Read the model definition and answer for the solid it produces. Units are mm, in the model's axes. A direction names the side the tool comes from. Coordinates: 2 decimals unless noted, no trailing zeros. Loops run counter-clockwise (first coordinate to the right, second up) from the corner with the lowest first, then second, coordinate; pieces in that order, holes last. Notation, with made-up numbers: M 65.5,84 L 104.5,84 A33 ccw 104.5,119 Z; hole C -13,8 d9. An arc over 180 degrees is marked long. One line per item, written item: value. Start each with the question number.
1. For faces 4 (the face through (-12.46, -83, 15)), 5 (the face through (13, -42, 30)), 6 (the face through (-15, -86, 15)), determine the directions among +Z, -Z, +X, -X, +Y, -Y from which every point of the face is accessible in a straight line to the end or side of a thin tool.
2. Flat-ended cylindrical pins translate along their axes: pin 1 (10 mm diameter, centred on x = -25.5, z = 20.5, fed in from -Y); pin 2 (3 mm diameter, centred on x = 19.5, z = 27, fed in from +Y); pin 3 (12.5 mm diameter, centred on x = -1.5, z = 9.5, fed in from +Y); pin 4 (5 mm diameter, centred on x = 32, z = 11.5, fed in from -Y). Find the tip coordinate at first contact, or state that the pin passes through.
3. The part is cut by section C-C (z = 6.75). Write down the section's boundary in (x, y), then the cut area to 3 significant figures.
4. The part is cut by section A-A (x = 0). Write down the section's boundary in (y, z), then the cut area to 3 significant figures.
5. The part is cut by section B-B (y = 0). Write down the section's boundary in (x, z), then the cut area to 3 significant figures.
6. Consider probe 1 along X at (y, z) = (0, 22); probe 2 along X at (y, z) = (-96, 3); probe 3 along Y at (x, z) = (6, 24.25). Determine where each line is inside the solid, lowest interval first.
7. Determine the mould class of faces 1 (the face through (0, -129.31, 15)), 2 (the face through (0, -126.77, 15)), 3 (the face through (15, -87, 15)) for opening direction Y: +Y half, -Y half, draft (parallel to the pull), parting line (faces both ways), or undercut.
```python
from build123d import *

# Parameters (mm, degrees)
F1_DEPTH = 30
F2_T     = -2.54


with BuildPart() as f1:
    # F0 (on Top) → F1 (new body)
    with BuildSketch(Plane.XY):
        with BuildLine():
            Line((15, -129.3097395662), (15, -42.9497395662))
            ThreePointArc((15, -42.9497395662), (0, 45.4937372481), (-15, -42.9497395662))
            Line((-15, -42.9497395662), (-15, -129.3097395662))
            Line((-15, -129.3097395662), (15, -129.3097395662))
        make_face()
    extrude(amount=F1_DEPTH)

    # F2
    f2_openings = [f1.faces().sort_by_distance(p)[0] for p in [
        (0, -24.43063, 30),
        (0, -24.43063, 0),
    ]]
    offset(amount=F2_T, openings=f2_openings, kind=Kind.INTERSECTION)


solid = f1.part
```
Answer block:
1. face 4: +Z, -Z
1. face 5: +Z, +X, -X, +Y, -Y
1. face 6: +Z, -Z, -X, -Y
2. pin 1: stops at y = -40.61
2. pin 2: stops at y = 41.78
2. pin 3: stops at y = 45.49
2. pin 4: stops at y = -34.63
3. outline: M -15,-129.31 L 15,-129.31 L 15,-42.95 A45.49 ccw long -15,-42.95 Z; hole M -12.46,-126.77 L 12.46,-126.77 L 12.46,-41.11 A42.95 ccw long -12.46,-41.11 Z
3. area: 1,140 mm2
4. outline: M -129.31,0 L -126.77,0 L -126.77,30 L -129.31,30 Z; M 42.95,0 L 45.49,0 L 45.49,30 L 42.95,30 Z
4. area: 152 mm2
5. outline: M -45.49,0 L -42.95,0 L -42.95,30 L -45.49,30 Z; M 42.95,0 L 45.49,0 L 45.49,30 L 42.95,30 Z
5. area: 152 mm2
6. probe 1: x = -45.49 to -42.95, 42.95 to 45.49
6. probe 2: x = -15 to -12.46, 12.46 to 15
6. probe 3: y = -129.31 to -126.77, 42.53 to 45.1
7. face 1: -Y half
7. face 2: undercut
7. face 3: draft
